The figure shows three views and two pictorial views of one solid part (mm, origin at its lowest corner). Answer the questions. Round coordinates to 2 decimals unless told otherwise and drop trailing zeros. Write each loop counter-clockwise with the first axis right and the second up, starting at its lowest first coordinate (ties: lowest second). Pieces come first, ordered by that corner, then holes. Notation, with made-up numbers: M 14.25,17 L 44.25,17 A14 ccw 44.25,37 Z; hole C 49.5,85 d6. An arc over 180 degrees is marked long. One line per item, written item: value. Start each with the question number.
Q1. Find section D-D (x = 26.5). Write down the section's boundary in (y, z), and give its area (3 significant figures).
Q2. Find section C-C (y = 7). Write down the section's boundary in (x, z), and give its area (3 significant figures).
Q3. The mould has two halves that part along Y. Classify the marked faces 1, 2 and 3: released by +Y, released by -Y, zero draft, split by the parting line, or undercut.
Q4. Find section A-A (z = 1.65). Write down the section's boundary in (x, y).
Q5. Find section B-B (x = 5). Write down the section's boundary in (y, z).
Q6. Consider probe 1 along X at (y, z) = (7, 1.65); probe 2 along Y at (x, z) = (5, 2); probe 3 along X at (y, z) = (7.5, 0.9). Determine where each line is inside the solid, lowest interval first.
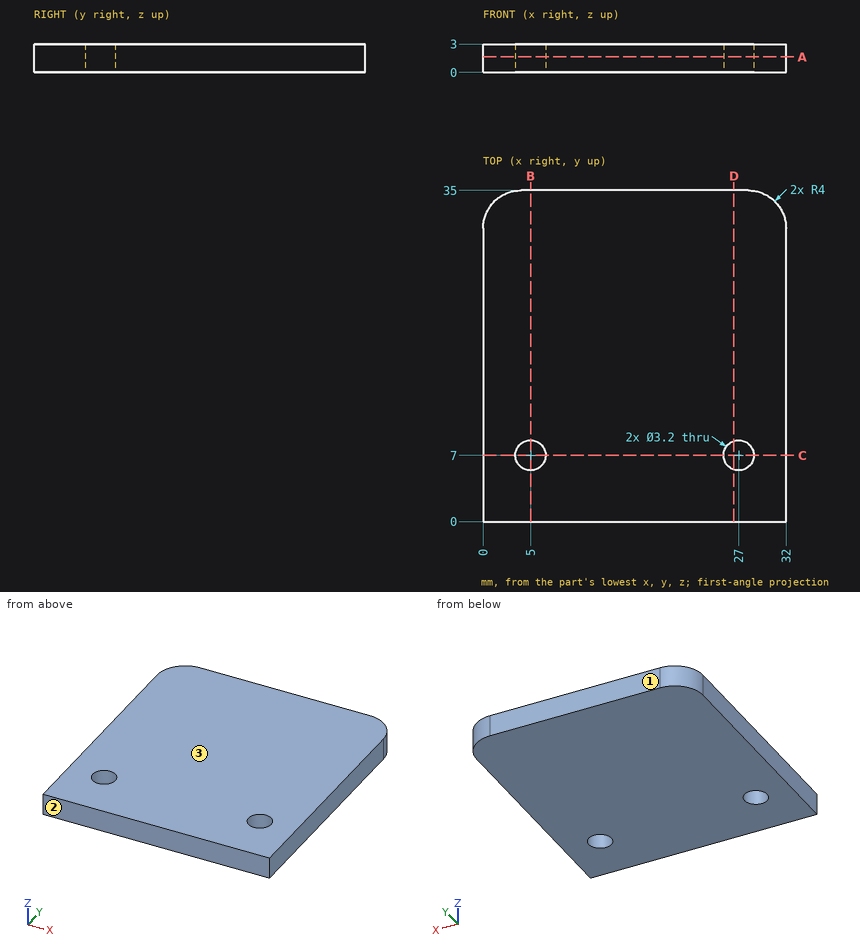
The answers:
1. outline: M 0,0 L 5.48,0 L 5.48,3 L 0,3 Z; M 8.52,0 L 35,0 L 35,3 L 8.52,3 Z
1. area: 95.9 mm2
2. outline: M 0,0 L 3.4,0 L 3.4,3 L 0,3 Z; M 6.6,0 L 25.4,0 L 25.4,3 L 6.6,3 Z; M 28.6,0 L 32,0 L 32,3 L 28.6,3 Z
2. area: 76.8 mm2
3. face 1: released by +Y
3. face 2: released by -Y
3. face 3: zero draft
4. outline: M 0,0 L 32,0 L 32,31 A4 ccw 28,35 L 4,35 A4 ccw 0,31 Z; hole C 5,7 d3.2; hole C 27,7 d3.2
5. outline: M 0,0 L 5.4,0 L 5.4,3 L 0,3 Z; M 8.6,0 L 35,0 L 35,3 L 8.6,3 Z
6. probe 1: 0 to 3.4, 6.6 to 25.4, 28.6 to 32
6. probe 2: 0 to 5.4, 8.6 to 35
6. probe 3: 0 to 3.48, 6.52 to 25.48, 28.52 to 32
